Part model, mm, in its own coordinate system. Face numbers are marked on the shaded views. A direction names the side the tool comes from. Give positions to 0.01 mm unless a question says otherwise; leave off trailing zeros. Loops run counter-clockwise (first coordinate to the right, second up) from the corner with the lowest first, then second, coordinate; pieces in that order, holes last. Notation, with made-up numbers: (-14.75, -12) -> (0.25, -12) arc R13 ccw to (0.25, 4) -> close; hole circle Ø3 at (43, 39). An arc over 180 degrees is marked (long way). One line per question, with ' | ' between items.
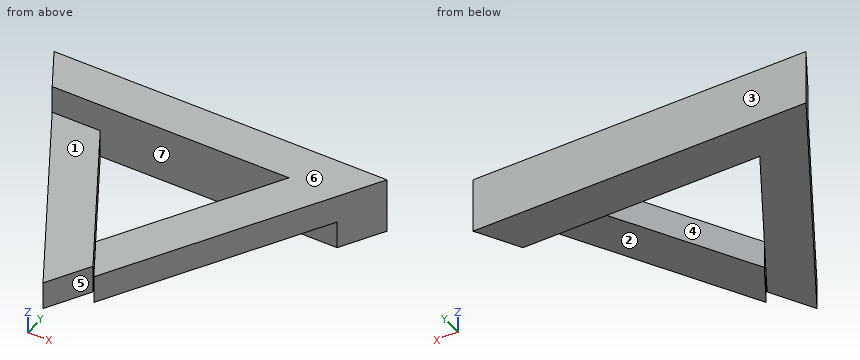
```python
from build123d import *

# Parameters (mm, degrees)
F1_DEPTH  = 10
F3_DEPTH  = 10.001
F7_DEPTH  = 10.001
F8_DEPTH  = 10.001
F9_DEPTH  = 5
F10_DEPTH = 5


with BuildPart() as f1:
    # F0 (on Top) → F1 (new body)
    with BuildSketch(Plane.XY):
        Polygon((30, 17.320508), (-30, 17.320508), (0, -34.641016), align=None)
    extrude(amount=F1_DEPTH)

    # F2 (on face) → F3 (cut, through all)
    with BuildSketch(Plane.XY.offset(10)):
        Polygon((17.009619, 9.820508), (-17.009619, 9.820508), (0, -19.641016), align=None)
    extrude(amount=-F3_DEPTH, mode=Mode.SUBTRACT)

    # F6 (on face) → F7 (cut, through all)
    with BuildSketch(Plane(origin=(0, 0, 0), x_dir=(1, 0, 0), z_dir=(0, 0, -1))):
        Polygon((4.330127, 27.141016), (0, 34.641016), (0, 19.641016), (0.25, 19.208003), (4.580127, 26.708003), align=None)
        Polygon((0, 19.641016), (0, 34.641016), (-4.330127, 27.141016), (-4.580127, 26.708003), (-0.25, 19.208003), align=None)
        Polygon((0.25, 19.208003), (0, 19.641016), (-0.25, 19.208003), align=None)
    extrude(amount=-F7_DEPTH, mode=Mode.SUBTRACT)

    # F6 (on face) → F8 (cut, through all)
    with BuildSketch(Plane(origin=(0, 0, 0), x_dir=(1, 0, 0), z_dir=(0, 0, -1))):
        Polygon((4.330127, 27.141016), (0, 34.641016), (0, 19.641016), (0.25, 19.208003), (4.580127, 26.708003), align=None)
        Polygon((0, 19.641016), (0, 34.641016), (-4.330127, 27.141016), (-4.580127, 26.708003), (-0.25, 19.208003), align=None)
        Polygon((0.25, 19.208003), (0, 19.641016), (-0.25, 19.208003), align=None)
    extrude(amount=-F8_DEPTH, mode=Mode.SUBTRACT)

    # F5 (on face) → F9 (cut)
    with BuildSketch(Plane.XY.offset(10)):
        Polygon((0, -34.641016), (0, -19.641016), (-17.009619, 9.820508), (-25.669873, 9.820508), align=None)
    extrude(amount=-F9_DEPTH, mode=Mode.SUBTRACT)

    # F4 (on face) → F10 (cut)
    with BuildSketch(Plane(origin=(0, 0, 0), x_dir=(1, 0, 0), z_dir=(0, 0, -1))):
        Polygon((0, 34.641016), (0, 19.641016), (17.009619, -9.820508), (25.669873, -9.820508), align=None)
    extrude(amount=-F10_DEPTH, mode=Mode.SUBTRACT)


solid = f1.part
```
1) Saw through at A-A (y = -6.5). Give the cut face in (x, z).
Found:
outline: (-16.25, 0) -> (-7.59, 0) -> (-7.59, 5) -> (-16.25, 5) -> close; (7.59, 5) -> (16.25, 5) -> (16.25, 10) -> (7.59, 10) -> close
2) Pin check, flat tips, straight feed: P1, Ø6, axis at y = -4, z = 3, coming from the -X side; P2, Ø4, axis at x = -2, z = 4, coming from the -Y side; P3, Ø5, axis at x = -11.5, z = 3.5, coming from the -Y side. Stop position of each tip, or through.
Found:
P1: x = -19.42 | P2: y = -25.7 | P3: y = -19.05
3) Tool access for the marked faces 1, 2 and 3: list every direction of +Z, -Z, +X, -X, +Y, -Y with a clear straight run to the whole face (end or side of a thin tool).
Found:
face 1: +Z, -X, -Y | face 2: -Z, +X, -Y | face 3: +Z, -Z, +X, -X, +Y
4) Pull direction Y, two halves, no side cores. Call the marked faces 4, 5, 6 and 7: pulls with the +Y half, pulls with the -Y half, needs draft (parallel to the pull), parting line crosses it, or undercut.
Found:
face 4: undercut | face 5: pulls with the -Y half | face 6: needs draft | face 7: undercut
5) Saw through at C-C (z = 8.25). Give the cut face in (x, y).
Found:
outline: (-30, 17.32) -> (-25.67, 9.82) -> (17.01, 9.82) -> (0.25, -19.21) -> (4.58, -26.71) -> (30, 17.32) -> close
6) Saw through at D-D (x = 20). Give the cut face in (y, z), and give its area (3 significant figures).
Found:
outline: (0, 5) -> (9.82, 5) -> (9.82, 0) -> (17.32, 0) -> (17.32, 10) -> (0, 10) -> close | area: 124 mm2
7) Saw through at B-B (x = 3). Give the cut face in (y, z), and give its area (3 significant figures).
Found:
outline: (-23.97, 5) -> (-14.44, 5) -> (-14.44, 10) -> (-23.97, 10) -> close; (9.82, 0) -> (17.32, 0) -> (17.32, 10) -> (9.82, 10) -> close | area: 123 mm2
8) Drill centre lines: line 1 (Z direction, x = -13.5, y = 3.5); line 2 (Y direction, x = -17, z = 5.5); line 3 (Y direction, x = -9, z = 4). Where is each one in solid material? Low to high.
Found:
line 1: 0 to 5 | line 2: 9.82 to 17.32 | line 3: -19.05 to -4.05, 9.82 to 17.32
